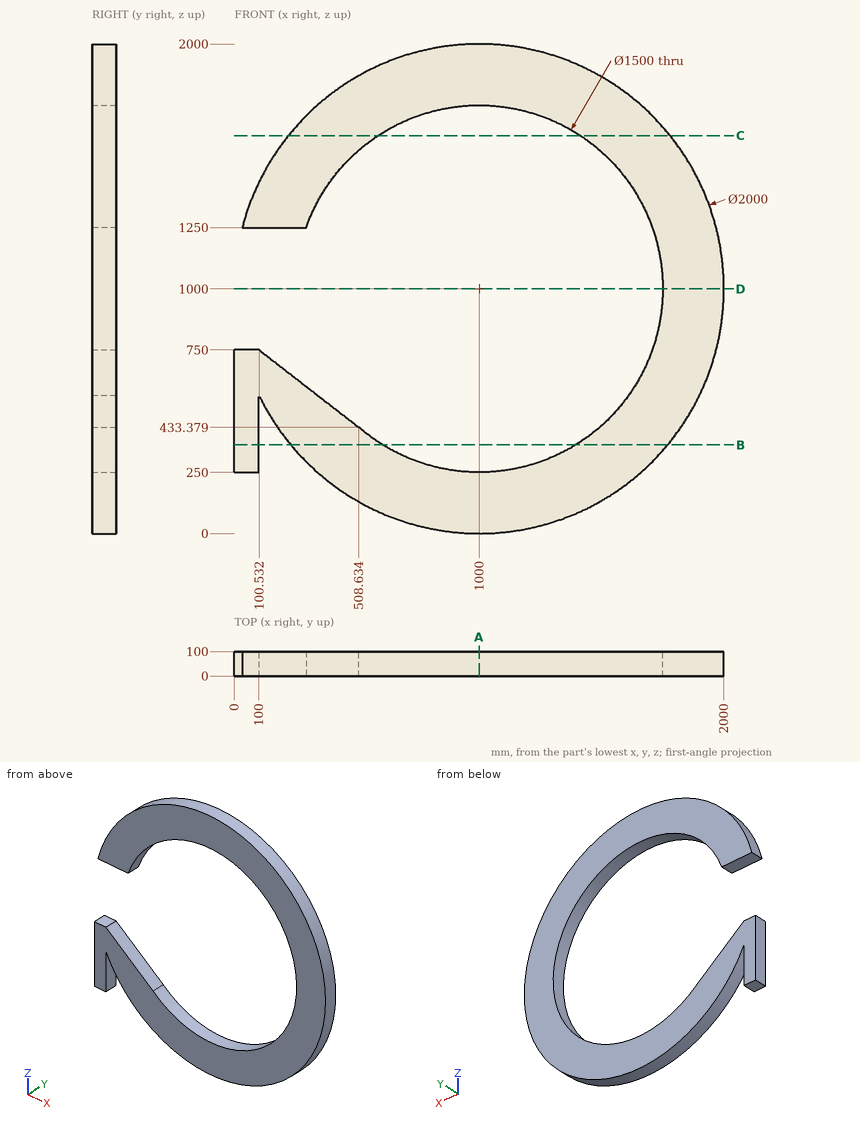
Part print with two shaded views. Sizes in mm from the minimum x, y, z corner. Give positions to 0.01 mm unless a question says otherwise; leave off trailing zeros. Order: outer loops, then holes, each group sorted by start corner. A loop starts at its lowest first (then second) coordinate and runs counter-clockwise, first axis right, second up. Notation, with made-up numbers: M -16.5,38.25 L 40.5,38.25 A19 ccw 40.5,47.25 Z; hole C 33.25,-14.75 d8. An arc over 180 degrees is marked long. Put each result on its own line as item: value.
Item 1: Cut at A-A on x = 1000. Write the cut outline in (y, z), then the cut area to 3 significant figures.
Results are:
outline: M 0,0 L 100,0 L 100,250 L 0,250 Z; M 0,1750 L 100,1750 L 100,2000 L 0,2000 Z
area: 50,000 mm2
Item 2: Wall check: probe 1 along Z at (x, y) = (1000, 56.5); probe 2 along X at (y, z) = (22.5, 560.5) (1 decimal); probe 3 along X at (y, z) = (44.5, 468) (1 decimal). Give the ranges that are in metal, low to high.
Results are:
probe 1: 0 to 250, 1750 to 2000
probe 2: 0 to 100, 101.8 to 344.8, 1607.7 to 1898.2
probe 3: 0 to 100, 153.3 to 464, 1528.7 to 1846.7
Item 3: Cut at C-C on z = 1626. Write the cut outline in (x, y).
Results are:
outline: M 220.18,0 L 586.93,0 L 586.93,100 L 220.18,100 Z; M 1413.07,0 L 1779.82,0 L 1779.82,100 L 1413.07,100 Z
Item 4: Drop flat-ended pins along their axis: pin 1 Ø1 at (y, z) = (44, 800) entering from -X; pin 2 Ø1 at (x, y) = (1629.5, 52.5) entering from +Z (1 decimal); pin 3 Ø12 at (x, y) = (741.5, 83) entering from -Z. Give the stop position or say it passes through.
Results are:
pin 1: x = 1722.7
pin 2: z = 1777.4
pin 3: z = 32.4
Item 5: Cut at B-B on z = 362. Write the cut outline in (x, y).
Results are:
outline: M 0,0 L 100,0 L 100,100 L 0,100 Z; M 229.96,0 L 605.72,0 L 605.72,100 L 229.96,100 Z; M 1394.28,0 L 1770.04,0 L 1770.04,100 L 1394.28,100 Z
Item 6: Cut at D-D on z = 1000. Write the cut outline in (x, y).
Results are:
outline: M 1750,0 L 2000,0 L 2000,100 L 1750,100 Z
